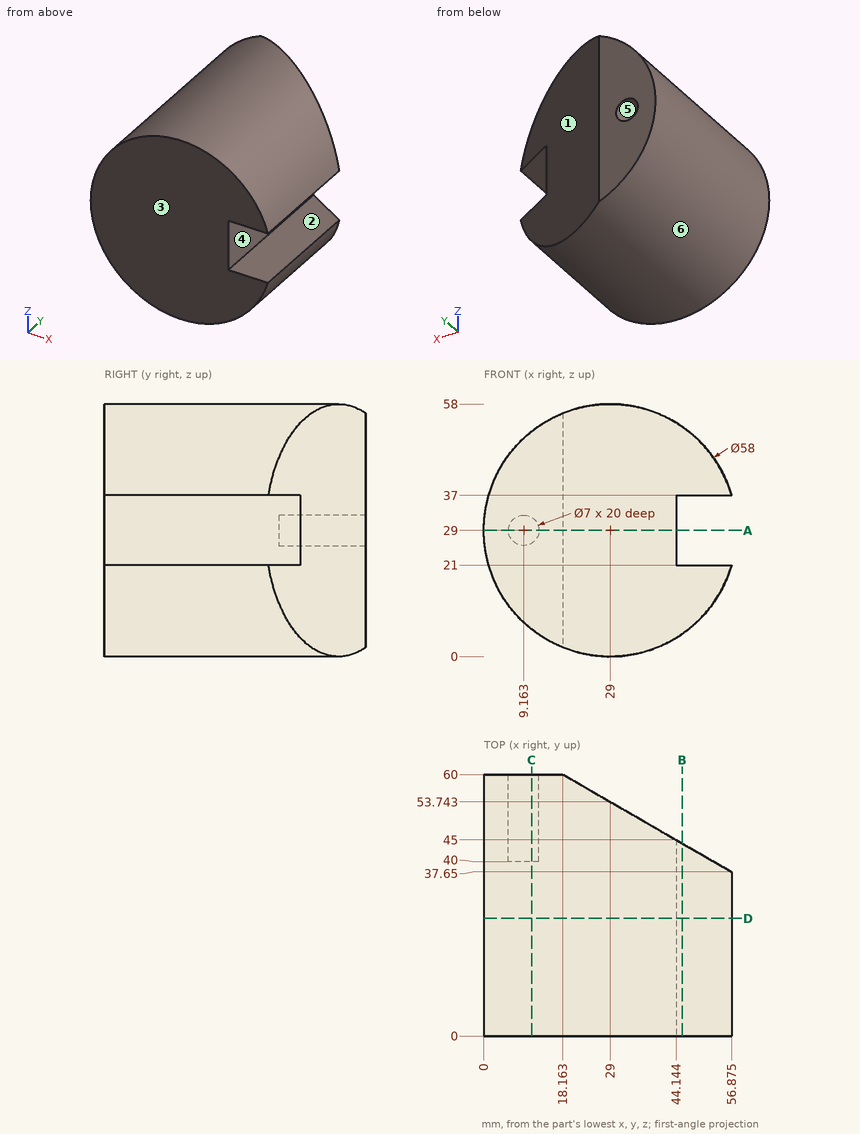
Design review of the part shown in the three views and the two pictorial views. Dimensions are in mm from the part's minimum x, y and z. A direction names the side the tool comes from. Give positions to 0.01 mm unless a question says otherwise; leave off trailing zeros. Write each loop counter-clockwise with the first axis right and the second up, starting at its lowest first coordinate (ties: lowest second). Pieces come first, ordered by that corner, then holes. Notation, with made-up numbers: M 5.5,84 L 18.5,84 A16 ccw 18.5,98 Z; hole C 70.5,62.25 d2. An arc over 180 degrees is marked long. One line per item, written item: value.
1) For line 1 (Z direction, x = 54.5, y = 7); line 2 (X direction, y = 54.75, z = 29) (1 decimal); line 3 (Z direction, x = 51.5, y = 13.5) (1 decimal), list the stretches that pass through material, from the lowest coordinate up. Write a range as from..to.
Results are:
line 1: z = 15.19..21, 37..42.81
line 2: x = 0..5.7, 12.7..27.3
line 3: z = 10.7..21, 37..47.3
2) For P1, Ø5, axis at y = 18.5, z = 7.5, coming from the -X side; P2, Ø1, axis at x = 40.5, y = 35, coming from the -Z side; P3, Ø4, axis at x = 53, y = 28.5, coming from the +Z side (1 decimal), all flat-tipped, find the tip position at first contact; note any pin that passes through.
Results are:
P1: stops at x = 7.09
P2: stops at z = 2.17
P3: stops at z = 47.9
3) Take a section at C-C, the plane x = 11. Write out the cut boundary in (y, z), then the cut area to 3 significant figures.
Results are:
outline: M 0,6.26 L 60,6.26 L 60,26.02 L 40,26.02 L 40,31.98 L 60,31.98 L 60,51.74 L 0,51.74 Z
area: 2,610 mm²
4) For the marked faces 1 and 2, list the 3-axis set-ups (+Z, -Z, +X, -X, +Y, -Y) from which the entire face can be reached by the end or side of a thin tool; tool diameter is ignored.
Results are:
face 1: +Z, -Z, +X, +Y
face 2: +X, +Y, -Y
5) The part is to be moulded in two halves that separate along Z. For the marked faces 3, 4, 5 and 6, say which applies: +Z half, -Z half, draft (parallel to the pull), parting line (faces both ways), or undercut.
Results are:
face 3: draft
face 4: undercut
face 5: undercut
face 6: parting line
6) Take a section at D-D, the plane y = 27. Write out the cut boundary in (x, z) (1 decimal), then the cut area to 3 significant figures.
Results are:
outline: M 44.1,21 L 44.1,37 L 56.9,37 A29 ccw long 56.9,21 Z
area: 2,430 mm²
7) Take a section at B-B, the plane x = 45.5. Write out the cut boundary in (y, z), then the cut area to 3 significant figures.
Results are:
outline: M 0,5.15 L 44.22,5.15 L 44.22,21 L 0,21 Z; M 0,37 L 44.22,37 L 44.22,52.85 L 0,52.85 Z
area: 1,400 mm²
8) Take a section at A-A, the plane z = 29. Write out the cut boundary in (x, y).
Results are:
outline: M 0,0 L 44.14,0 L 44.14,45 L 18.16,60 L 12.66,60 L 12.66,40 L 5.66,40 L 5.66,60 L 0,60 Z
